Source: CAD feature listing. Evaluate the final solid. Frame: model axes, mm. Face numbers are marked on the shaded views. A direction names the side the tool comes from. Give positions to 0.01 mm unless a question says otherwise; leave off trailing zeros. Write each loop counter-clockwise with the first axis right and the second up, starting at its lowest first coordinate (ties: lowest second). Pieces come first, ordered by that corner, then holes.
```python
from build123d import *

# Parameters (mm, degrees)
SKETCH1_R                                           = 5
BOSS_EXTRUDE1_DEPTH                                 = 15
SKETCH2_R                                           = 27
SKETCH2_R_2                                         = 17
CUT_EXTRUDE_THIN1_DEPTH                             = 8
CBORE_FOR_M4_HEX_SOCKET_HEAD_CAP_SCREW1_D           = 4.3
CBORE_FOR_M4_HEX_SOCKET_HEAD_CAP_SCREW1_DEPTH       = 8.5
CBORE_FOR_M4_HEX_SOCKET_HEAD_CAP_SCREW1_CBORE_D     = 8
CBORE_FOR_M4_HEX_SOCKET_HEAD_CAP_SCREW1_CBORE_DEPTH = 4.4
CBORE_FOR_M4_HEX_SOCKET_HEAD_CAP_SCREW1_TIP         = 1.291850331
CBORE_FOR_M4_HEX_SOCKET_HEAD_CAP_SCREW2_D           = 4.3
CBORE_FOR_M4_HEX_SOCKET_HEAD_CAP_SCREW2_DEPTH       = 8.5
CBORE_FOR_M4_HEX_SOCKET_HEAD_CAP_SCREW2_CBORE_D     = 8
CBORE_FOR_M4_HEX_SOCKET_HEAD_CAP_SCREW2_CBORE_DEPTH = 4.4
CBORE_FOR_M4_HEX_SOCKET_HEAD_CAP_SCREW2_TIP         = 1.291850331
CBORE_FOR_M4_HEX_SOCKET_HEAD_CAP_SCREW3_D           = 4.3
CBORE_FOR_M4_HEX_SOCKET_HEAD_CAP_SCREW3_DEPTH       = 8.5
CBORE_FOR_M4_HEX_SOCKET_HEAD_CAP_SCREW3_CBORE_D     = 8
CBORE_FOR_M4_HEX_SOCKET_HEAD_CAP_SCREW3_CBORE_DEPTH = 4.4
CBORE_FOR_M4_HEX_SOCKET_HEAD_CAP_SCREW3_TIP         = 1.291850331
CBORE_FOR_M4_HEX_SOCKET_HEAD_CAP_SCREW4_D           = 4.3
CBORE_FOR_M4_HEX_SOCKET_HEAD_CAP_SCREW4_DEPTH       = 8.5
CBORE_FOR_M4_HEX_SOCKET_HEAD_CAP_SCREW4_CBORE_D     = 8
CBORE_FOR_M4_HEX_SOCKET_HEAD_CAP_SCREW4_CBORE_DEPTH = 4.4
CBORE_FOR_M4_HEX_SOCKET_HEAD_CAP_SCREW4_TIP         = 1.291850331


with BuildPart() as part:
    # Sketch1 → Boss-Extrude1 (new body)
    with BuildSketch(Plane.XY):
        with BuildLine():
            Line((15.329709717, -21), (-15.329709717, -21))
            ThreePointArc((-15.329709717, -21), (-18.384776311, -18.384776311), (-21, -15.329709717))
            Line((-21, -15.329709717), (-21, 15.329709717))
            ThreePointArc((-21, 15.329709717), (-18.384776311, 18.384776311), (-15.329709717, 21))
            Line((-15.329709717, 21), (15.329709717, 21))
            ThreePointArc((15.329709717, 21), (18.384776311, 18.384776311), (21, 15.329709717))
            Line((21, 15.329709717), (21, -15.329709717))
            ThreePointArc((21, -15.329709717), (18.384776311, -18.384776311), (15.329709717, -21))
        make_face()
        Circle(SKETCH1_R, mode=Mode.SUBTRACT)
    extrude(amount=BOSS_EXTRUDE1_DEPTH)

    # Sketch2 → Cut-Extrude-Thin1 (cut)
    with BuildSketch(Plane.XY.offset(15)):
        Circle(SKETCH2_R)
        Circle(SKETCH2_R_2, mode=Mode.SUBTRACT)
    extrude(amount=-CUT_EXTRUDE_THIN1_DEPTH, mode=Mode.SUBTRACT)

    # CBORE for M4 Hex Socket Head Cap Screw1
    with Locations(Plane(origin=(-14.849242405, 14.849242405, 0), x_dir=(-1, 0, 0), z_dir=(0, 0, -1))):
        with Locations((0, 0)):
            CounterBoreHole(CBORE_FOR_M4_HEX_SOCKET_HEAD_CAP_SCREW1_D / 2, CBORE_FOR_M4_HEX_SOCKET_HEAD_CAP_SCREW1_CBORE_D / 2, CBORE_FOR_M4_HEX_SOCKET_HEAD_CAP_SCREW1_CBORE_DEPTH, depth=CBORE_FOR_M4_HEX_SOCKET_HEAD_CAP_SCREW1_DEPTH)
            with Locations((0, 0, -(CBORE_FOR_M4_HEX_SOCKET_HEAD_CAP_SCREW1_DEPTH + CBORE_FOR_M4_HEX_SOCKET_HEAD_CAP_SCREW1_TIP / 2))):  # 118° drill point
                Cone(0, CBORE_FOR_M4_HEX_SOCKET_HEAD_CAP_SCREW1_D / 2, CBORE_FOR_M4_HEX_SOCKET_HEAD_CAP_SCREW1_TIP, mode=Mode.SUBTRACT)

    # CBORE for M4 Hex Socket Head Cap Screw2
    with Locations(Plane(origin=(14.849242405, 14.849242405, 0), x_dir=(-1, 0, 0), z_dir=(0, 0, -1))):
        with Locations((0, 0)):
            CounterBoreHole(CBORE_FOR_M4_HEX_SOCKET_HEAD_CAP_SCREW2_D / 2, CBORE_FOR_M4_HEX_SOCKET_HEAD_CAP_SCREW2_CBORE_D / 2, CBORE_FOR_M4_HEX_SOCKET_HEAD_CAP_SCREW2_CBORE_DEPTH, depth=CBORE_FOR_M4_HEX_SOCKET_HEAD_CAP_SCREW2_DEPTH)
            with Locations((0, 0, -(CBORE_FOR_M4_HEX_SOCKET_HEAD_CAP_SCREW2_DEPTH + CBORE_FOR_M4_HEX_SOCKET_HEAD_CAP_SCREW2_TIP / 2))):  # 118° drill point
                Cone(0, CBORE_FOR_M4_HEX_SOCKET_HEAD_CAP_SCREW2_D / 2, CBORE_FOR_M4_HEX_SOCKET_HEAD_CAP_SCREW2_TIP, mode=Mode.SUBTRACT)

    # CBORE for M4 Hex Socket Head Cap Screw3
    with Locations(Plane(origin=(14.849242405, -14.849242405, 0), x_dir=(-1, 0, 0), z_dir=(0, 0, -1))):
        with Locations((0, 0)):
            CounterBoreHole(CBORE_FOR_M4_HEX_SOCKET_HEAD_CAP_SCREW3_D / 2, CBORE_FOR_M4_HEX_SOCKET_HEAD_CAP_SCREW3_CBORE_D / 2, CBORE_FOR_M4_HEX_SOCKET_HEAD_CAP_SCREW3_CBORE_DEPTH, depth=CBORE_FOR_M4_HEX_SOCKET_HEAD_CAP_SCREW3_DEPTH)
            with Locations((0, 0, -(CBORE_FOR_M4_HEX_SOCKET_HEAD_CAP_SCREW3_DEPTH + CBORE_FOR_M4_HEX_SOCKET_HEAD_CAP_SCREW3_TIP / 2))):  # 118° drill point
                Cone(0, CBORE_FOR_M4_HEX_SOCKET_HEAD_CAP_SCREW3_D / 2, CBORE_FOR_M4_HEX_SOCKET_HEAD_CAP_SCREW3_TIP, mode=Mode.SUBTRACT)

    # CBORE for M4 Hex Socket Head Cap Screw4
    with Locations(Plane(origin=(-14.849242405, -14.849242405, 0), x_dir=(-1, 0, 0), z_dir=(0, 0, -1))):
        with Locations((0, 0)):
            CounterBoreHole(CBORE_FOR_M4_HEX_SOCKET_HEAD_CAP_SCREW4_D / 2, CBORE_FOR_M4_HEX_SOCKET_HEAD_CAP_SCREW4_CBORE_D / 2, CBORE_FOR_M4_HEX_SOCKET_HEAD_CAP_SCREW4_CBORE_DEPTH, depth=CBORE_FOR_M4_HEX_SOCKET_HEAD_CAP_SCREW4_DEPTH)
            with Locations((0, 0, -(CBORE_FOR_M4_HEX_SOCKET_HEAD_CAP_SCREW4_DEPTH + CBORE_FOR_M4_HEX_SOCKET_HEAD_CAP_SCREW4_TIP / 2))):  # 118° drill point
                Cone(0, CBORE_FOR_M4_HEX_SOCKET_HEAD_CAP_SCREW4_D / 2, CBORE_FOR_M4_HEX_SOCKET_HEAD_CAP_SCREW4_TIP, mode=Mode.SUBTRACT)


solid = part.part
```
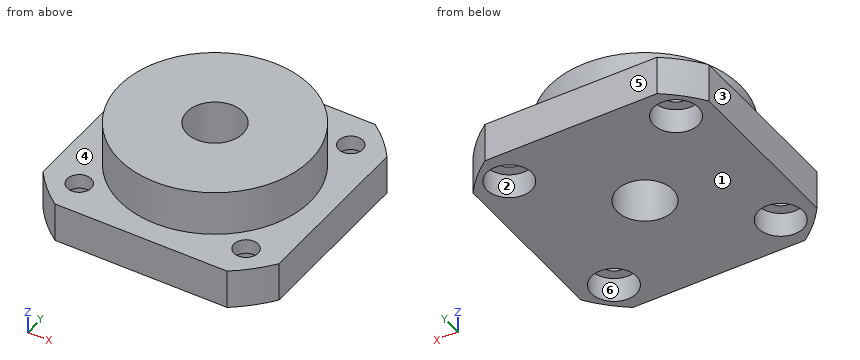
1. Section query C-C (z = 8.5). Return loops of the section in (x, y).
2. Pin query (flat end, axial travel): P1, Ø5, axis at x = 14.85, y = 14.85, coming from the -Z side; P2, Ø3, axis at y = 1.5, z = 12, coming from the -X side; P3, Ø7, axis at x = 14.85, y = -14.85, coming from the +Z side. Return the tip coordinate at first contact, or that it passes through.
3. Line query: probe 1 along Z at (x, y) = (18.5, -0.5); probe 2 along Y at (x, z) = (-4, 2); probe 3 along Y at (x, z) = (-3.5, 7.25). Output: solid intervals per line, ascending.
4. Pull-direction query (X, two-part tool) for the marked faces 1, 2 and 3; classes: pulls with the +X half, pulls with the -X half, needs draft (parallel to the pull), parting line crosses it, or undercut.
5. Section query A-A (x = 0). Return loops of the section in (y, z).
6. Section query D-D (y = 8). Return loops of the section in (x, z), plus the area to 3 significant figures.
7. Access query for the marked faces 4, 5 and 6. Directions: +Z, -Z, +X, -X, +Y, -Y. A direction counts if a zero-diameter tool reaches every point of the face in a straight line with its end or side. Return the directions, or none.
The answers:
1. outline: circle Ø34 at (0, 0); hole circle Ø10 at (0, 0)
2. P1: stops at z = 4.4
2. P2: stops at x = -17
2. P3: stops at z = 7
3. probe 1: z = 0 to 7
3. probe 2: y = -21 to -3, 3 to 21
3. probe 3: y = -16.64 to -3.57, 3.57 to 16.64
4. face 1: needs draft
4. face 2: undercut
4. face 3: pulls with the -X half
5. outline: (-21, 0) - (-5, 0) - (-5, 15) - (-17, 15) - (-17, 7) - (-21, 7) - close; (5, 0) - (21, 0) - (21, 7) - (17, 7) - (17, 15) - (5, 15) - close
6. outline: (-21, 0) - (21, 0) - (21, 7) - (15, 7) - (15, 15) - (-15, 15) - (-15, 7) - (-21, 7) - close
6. area: 534 mm2
7. face 4: +Z
7. face 5: +Z, -Z, +X, -X, +Y
7. face 6: -Z
